from build123d import *

# Parameters (mm, degrees)
COPIED_SKETCH_DONT_MESS_WITH_DEPTH = 3.175
SKETCH3_R                          = 3.175
HOLE_FOR_TOP_SUPPORT_BRACING_DEPTH = 4.175
SKETCH4_R                          = 3.175
MAKING_IT_MACHINABLE_DEPTH         = 4.175
SKETCH5_R                          = 2.6289
THING_FOR_HARDSTOP_DEPTH           = 3.175
FILLET1_R                          = 6.35
SKETCH6_R                          = 2.6289
CUT_EXTRUDE1_DEPTH                 = 4.175


with BuildPart() as part:
    # Sketch2 → Copied sketch - dont mess with (new body)
    with BuildSketch(Plane.XY):
        with BuildLine():
            Line((155.660230842, 130.614442288), (160.524613056, 134.69614361))
            ThreePointArc((160.524613056, 134.69614361), (200.900960932, 59.581930119), (208.004909798, -25.4))
            Line((208.004909798, -25.4), (225.775729431, -25.4))
            ThreePointArc((225.775729431, -25.4), (217.513785946, 65.632255207), (174.045297477, 146.041344921))
            Line((174.045297477, 146.041344921), (139.503343029, 159.851365822))
            ThreePointArc((139.503343029, 159.851365822), (129.618020291, 158.107153482), (126.784391338, 148.47738561))
            Line((126.784391338, 148.47738561), (136.202701987, 114.287637002))
            ThreePointArc((136.202701987, 114.287637002), (167.077347976, 60.811181483), (177.8, 0))
            Line((177.8, 0), (177.8, -25.4))
            Line((177.8, -25.4), (201.606249903, -25.4))
            ThreePointArc((201.606249903, -25.4), (194.922962004, 57.404519712), (155.660230842, 130.614442288))
        make_face()
    extrude(amount=COPIED_SKETCH_DONT_MESS_WITH_DEPTH)

    # Sketch3 → Hole for top support bracing (cut, through all)
    with BuildSketch(Plane.XY.offset(3.175)):
        with Locations((135.967339212, 151.007028537)):
            Circle(SKETCH3_R)
    extrude(amount=-HOLE_FOR_TOP_SUPPORT_BRACING_DEPTH, mode=Mode.SUBTRACT)

    # Sketch4 → Making it machinable (cut, through all)
    with BuildSketch(Plane.XY.offset(3.175)):
        with Locations((158.092421949, 132.655292949)):
            Circle(SKETCH4_R)
    extrude(amount=-MAKING_IT_MACHINABLE_DEPTH, mode=Mode.SUBTRACT)

    # Sketch5 → Thing for hardstop (add)
    with BuildSketch(Plane.XY.offset(3.175)):
        with BuildLine():
            Line((225.775729431, -25.4), (236.774252059, -31.75))
            ThreePointArc((236.774252059, -31.75), (245.448513373, -29.425738686), (243.124252059, -20.751477372))
            Line((243.124252059, -20.751477372), (226.914188257, -11.392592672))
            ThreePointArc((226.914188257, -11.392592672), (226.453289353, -18.405100951), (225.775729431, -25.4))
        make_face()
        with Locations((239.949252059, -26.250738686)):
            Circle(SKETCH5_R, mode=Mode.SUBTRACT)
    extrude(amount=-THING_FOR_HARDSTOP_DEPTH)

    # Fillet1
    fillet1_edges = [part.edges().sort_by_distance(p)[0] for p in [
        (226.914188257, -11.392592672, 1.5875),
    ]]
    fillet(fillet1_edges, radius=FILLET1_R)

    # Sketch6 → Cut-Extrude1 (cut, through all)
    with BuildSketch(Plane.XY.offset(3.175)):
        with Locations((147.764763317, 140.384580161)):
            Circle(SKETCH6_R)
    extrude(amount=-CUT_EXTRUDE1_DEPTH, mode=Mode.SUBTRACT)


solid = part.part
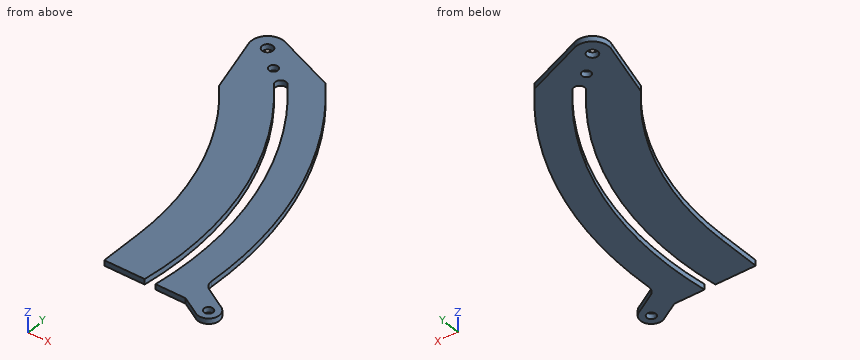
Work out the finished part from the listing and answer in its coordinate system (mm). Round coordinates to 2 decimals unless told otherwise and drop trailing zeros. Write each loop counter-clockwise with the first axis right and the second up, starting at its lowest first coordinate (ties: lowest second). Pieces come first, ordered by that corner, then holes. Notation, with made-up numbers: (-23, 9) - (17, 9) arc R8 cw to (17, 20) - close; hole circle Ø8 at (9.5, 22). An arc over 180 degrees is marked (long way). Answer in a Markdown table with one row per item. Add a question column.
1. A cutting plane is placed at C-C, the plane z = 0.55. Determine the outline of the cut face in (x, y) (3 decimals), and give its area (3 significant figures).
2. Given pin 1 (1.6 mm diameter, centred on x = 216, z = 2, fed in from -Y), flat-ended and moving along its own axis, determine where the tip first touches the part or whether it passes through.
3. A cutting plane is placed at A-A, the plane y = 43. Determine the outline of the cut face in (x, z) (3 decimals), and give its area (3 significant figures).
4. A cutting plane is placed at D-D, the plane x = 220.5. Determine the outline of the cut face in (y, z) (3 decimals).
5. A cutting plane is placed at B-B, the plane x = 165. Determine the outline of the cut face in (y, z) (3 decimals).
6. Find the intervals of material crossed by line 1 along X through (y, z) = (-6.5, 1.75); line 2 along X through (y, z) = (25, 2.3); line 3 along Y through (x, z) = (183.5, 0.3), in increasing order. Write a range as from..to.
Worked out:
| question | item | result |
|---|---|---|
| 1 | outline | (126.784, 148.477) - (136.203, 114.288) arc R177.8 cw to (177.8, 0) - (177.8, -25.4) - (201.606, -25.4) arc R203.2 ccw to (155.66, 130.614) arc R3.175 cw to (160.525, 134.696) arc R209.55 cw to (208.005, -25.4) - (225.776, -25.4) - (236.774, -31.75) arc R6.35 ccw to (243.124, -20.751) - (230.244, -13.315) arc R6.35 cw to (227.073, -7.603) arc R227.2 ccw to (174.045, 146.041) - (139.503, 159.851) arc R9.525 ccw to start; hole circle Ø6.35 at (135.967, 151.007); hole circle Ø5.258 at (147.765, 140.385); hole circle Ø5.258 at (239.949, -26.251) |
| 1 | area | 8,470 mm^2 |
| 2 | pin 1 | y = -25.4 |
| 3 | outline | (172.522, 0) - (198.598, 0) - (198.598, 3.175) - (172.522, 3.175) - close; (205.091, 0) - (223.094, 0) - (223.094, 3.175) - (205.091, 3.175) - close |
| 3 | area | 140 mm^2 |
| 4 | outline | (-25.4, 0) - (54.769, 0) - (54.769, 3.175) - (-25.4, 3.175) - close |
| 5 | outline | (66.241, 0) - (118.597, 0) - (118.597, 3.175) - (66.241, 3.175) - close; (129.175, 0) - (149.658, 0) - (149.658, 3.175) - (129.175, 3.175) - close |
| 6 | line 1 | 177.8..203.1, 209.45..227.11 |
| 6 | line 2 | 176.03..201.66, 208.05..225.82 |
| 6 | line 3 | -25.4..87.28, 101.19..133.97 |
